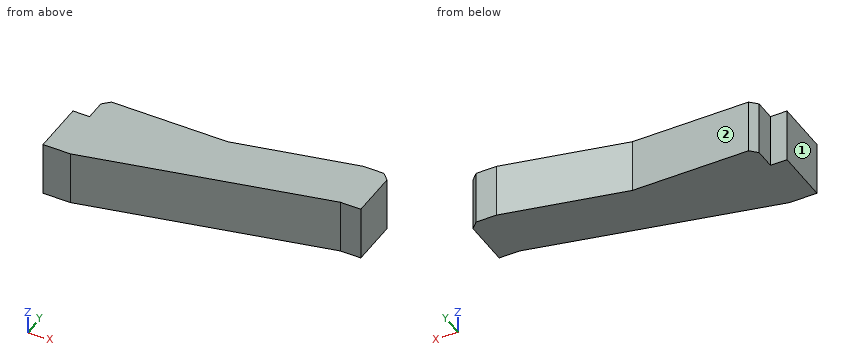
from build123d import *

# Parameters (mm, degrees)
BOSS_EXTRUDE1_DEPTH = 1.984375
CHAMFER1_SIZE       = 0.25


with BuildPart() as part:
    # Sketch1 → Boss-Extrude1 (new body)
    with BuildSketch(Plane.XY):
        Polygon((0, 0), (1, 0), (1, -1.984375), (0.25, -1.984375), (-8.526125475, -3.96875), (-9.526125475, -3.96875), (-9.526125475, -1.984375), (-8.92, -1.984375), (-8.92, -0.984375), (-4.42488189, -0.984375), align=None)
    extrude(amount=BOSS_EXTRUDE1_DEPTH)

    # Chamfer1
    chamfer1_edges = [part.edges().sort_by_distance(p)[0] for p in [
        (1, 0, 0.9921875),
        (-8.92, -0.984375, 0.9921875),
    ]]
    chamfer(chamfer1_edges, length=CHAMFER1_SIZE)


solid = part.part
Can you work these out from the model? Positions are in its coordinate system, mm. Face numbers are marked on the shaded views. A direction names the side the tool comes from. Give positions to 0.01 mm unless a question says otherwise; leave off trailing zeros. Order: outer loops, then holes, each group sorted by start corner. A loop starts at its lowest first (then second) coordinate and runs counter-clockwise, first axis right, second up. Notation, with made-up numbers: M 17.25,83.25 L 72.25,83.25 A23 cw 72.25,115.25 Z; hole C 50,67 d11. An arc over 180 degrees is marked long. Use a Markdown table: item, result. Add a question column.
Item 1: For the marked faces 1 and 2, which set-ups out of +Z, -Z, +X, -X, +Y, -Y let a thin tool reach every point of the face, with its end or its side?
Item 2: Suppose I cut it at C-C (x = -5.5). List the corners of the cut face in (y, z) for me.
Item 3: If I drill on L1, parallel to Y at x = -1, z = 1.45; L2, parallel to X at y = -1.1, z = 0.15; L3, parallel to Y at x = -4.75, z = 0.2, over which ranges is the centre line in solid material (lowest first)? Write a range as [from, to].
Item 4: Will this pin go through, and if not, where does the flat tip stop? pin 1 (0.6 mm diameter, centred on y = -1.5, z = 1, fed in from -X).
Item 5: Suppose I cut it at A-A (z = 0.85). List the corners of the cut face in (x, y) for me, then the cut area to 3 significant figures.
Item 6: Suppose I cut it at B-B (y = -1.7). List the corners of the cut face in (x, z) for me, then the cut area to 3 significant figures.
Answer sheet:
| question | item | result |
|---|---|---|
| 1 | face 1 | +Z, -Z, -X, +Y, -Y |
| 1 | face 2 | +Z, -Z, -X, +Y |
| 2 | outline | M -3.28,0 L -0.98,0 L -0.98,1.98 L -3.28,1.98 Z |
| 3 | L1 | y = [-2.27, -0.22] |
| 3 | L2 | x = [-8.79, 1] |
| 3 | L3 | y = [-3.11, -0.98] |
| 4 | pin 1 | stops at x = -8.92 |
| 5 | outline | M -9.53,-3.97 L -8.53,-3.97 L 0.25,-1.98 L 1,-1.98 L 1,-0.25 L 0.75,0 L 0,0 L -4.42,-0.98 L -8.67,-0.98 L -8.92,-1.23 L -8.92,-1.98 L -9.53,-1.98 Z |
| 5 | area | 23.7 mm² |
| 6 | outline | M -8.92,0 L 1,0 L 1,1.98 L -8.92,1.98 Z |
| 6 | area | 19.7 mm² |
